```python
from build123d import *

# Parameters (mm, degrees)
F1_DEPTH       = 4.765
F4_D           = 5.5
F4_DEPTH       = 8
F4_TIP         = 1.6523667023
F4_ON_F3_D     = 5.5
F4_ON_F3_DEPTH = 8
F4_ON_F3_TIP   = 1.6523667023


with BuildPart() as f1:
    # F0 (on Right) → F1 (new body, symmetric)
    with BuildSketch(Plane.YZ):
        Polygon((-32, 0), (0, 0), (0, 290), (-10, 290), align=None)
    extrude(amount=F1_DEPTH, both=True)

    # F4
    with Locations(Plane(origin=(0, 0, 0), x_dir=(-1, 0, 0), z_dir=(0, 1, 0))):
        with Locations((0, 60), (0, 140), (0, 220)):
            Hole(F4_D / 2, depth=F4_DEPTH)
            with Locations((0, 0, -(F4_DEPTH + F4_TIP / 2))):  # 118° drill point
                Cone(0, F4_D / 2, F4_TIP, mode=Mode.SUBTRACT)

    # F4 on F3
    with Locations(Plane(origin=(0, 0, 0), x_dir=(1, 0, 0), z_dir=(0, 0, -1))):
        with Locations((0, 22), (0, 10)):
            Hole(F4_ON_F3_D / 2, depth=F4_ON_F3_DEPTH)
            with Locations((0, 0, -(F4_ON_F3_DEPTH + F4_ON_F3_TIP / 2))):  # 118° drill point
                Cone(0, F4_ON_F3_D / 2, F4_ON_F3_TIP, mode=Mode.SUBTRACT)


solid = f1.part
```
Model file for the job. Use its own axes, mm. A direction names the side the tool comes from. Coordinates: 2 decimals unless noted, no trailing zeros. Order: outer loops, then holes, each group sorted by start corner. A loop starts at its lowest first (then second) coordinate and runs counter-clockwise, first axis right, second up. Notation, with made-up numbers: (70.5, -16) -> (96.5, -16) arc R11 ccw to (96.5, 1) -> close; hole circle Ø1 at (18.25, 53). An arc over 180 degrees is marked (long way). Answer as a JSON object with one key per item and string values. Group by question number.
1) Flat gauge pins, fed straight in: pin 1 (2 mm diameter, centred on x = -3.5, z = 38, fed in from -Y); pin 2 (1.5 mm diameter, centred on x = -0.5, z = 223.5, fed in from -Y); pin 3 (1 mm diameter, centred on x = 1, z = 50, fed in from -Y). Where does each tip first touch, or does it go through?
2) Which spindle directions (+Z, -Z, +X, -X, +Y, -Y) get a long thin tool onto all of the face, cutting with end or side? Do faces 1 (the face through (-0.596, -4.056, 137.315)), 2 (the face through (0, -5, 290)), 3 (the face through (0.358, -12.727, 4.056)). Say none if no direction does.
3) Cut at A-A, the plane z = 228.5. Write the cut outline in (x, y) (3 decimals), then the cut area to 3 significant figures.
4) Pull direction Z, two halves, no side cores. Call faces 4 (the face through (0.358, -24.727, 4.056)), 5 (the face through (0.067, -20.846, 147.03)), 6 (the face through (-0.104, -21.534, 9.365)), 7 (the face through (0.06, -9.37, 220.47)): +Z half, -Z half, draft (parallel to the pull), parting line (faces both ways), or undercut.
5) Cut at B-B, the plane y = -27.5. Write the cut outline in (x, z) (3 decimals), then the cut area to 3 significant figures.
6) Drill centre lines: L1, parallel to Z at x = 0, y = -3; L2, parallel to X at y = -22, z = 6 (3 decimals); L3, parallel to Z at x = 0.5, y = -8.5. Where is each one in solid material? Low to high.
Check values:
{
 "1": {"pin 1": "stops at y = -29.19", "pin 2": "stops at y = -15.1", "pin 3": "stops at y = -28.24"},
 "2": {"face 1": "+Y", "face 2": "+Z, +X, -X, +Y, -Y", "face 3": "-Z"},
 "3": {"outline": "(-4.765, -14.666) -> (4.765, -14.666) -> (4.765, 0) -> (-4.765, 0) -> close", "area": "140 mm²"},
 "4": {"face 4": "draft", "face 5": "+Z half", "face 6": "-Z half", "face 7": "undercut"},
 "5": {"outline": "(-4.765, 0) -> (4.765, 0) -> (4.765, 59.318) -> (-4.765, 59.318) -> close", "area": "565 mm²"},
 "6": {"L1": "z = 0 to 57.25, 62.75 to 137.25, 142.75 to 217.25, 222.75 to 290", "L2": "x = -4.765 to -2.75, 2.75 to 4.765", "L3": "z = 8.7 to 58.15, 61.85 to 138.15, 141.85 to 218.15, 221.85 to 290"}
}
